Model file for the job. Use its own axes, mm. Face numbers are marked on the shaded views. A direction names the side the tool comes from. Coordinates: 2 decimals unless noted, no trailing zeros. Order: outer loops, then holes, each group sorted by start corner. A loop starts at its lowest first (then second) coordinate and runs counter-clockwise, first axis right, second up. Notation, with made-up numbers: M 4.25,-6.5 L 30.25,-6.5 A30 ccw 30.25,24.5 Z; hole C 54,38 d2. An arc over 180 degrees is marked long. Return JSON: item names as keys, results as strings.
```python
from build123d import *

# Parameters (mm, degrees)
F0_W     = 4.6228
F0_H     = 4.6228
F1_DEPTH = 3.175
F2_DEPTH = 34.925
F3_W     = 4.6228
F3_H     = 4.6228
F4_DEPTH = 25.4


with BuildPart() as f1:
    # F0 (on Front) → F1 (new body)
    with BuildSketch(Plane.XZ):
        Polygon((6.37921, -9.525), (6.37921, 15.875), (-6.37921, 15.875), (-6.37921, -9.525), (-1.8334548599, -9.525), align=None)
        with Locations((-0.02921, -3.175)):
            Rectangle(F0_W, F0_H, mode=Mode.SUBTRACT)
        with Locations((-0.02921, 9.525)):
            Rectangle(F0_W, F0_H, mode=Mode.SUBTRACT)
    extrude(amount=F1_DEPTH)

    # F0 (on Front) → F2 (join)
    with BuildSketch(Plane.XZ):
        Polygon((6.37921, -12.7), (6.37921, -9.525), (-1.8334548599, -9.525), (-6.37921, -9.525), (-6.37921, -12.7), (2.7123002801, -12.7), align=None)
    extrude(amount=F2_DEPTH)

    # F3 (on face) → F4 (cut)
    with BuildSketch(Plane.XY.offset(-9.525)):
        with Locations((0, -14.8336)):
            Rectangle(F3_W, F3_H)
        Polygon((-2.3114, -30.8864), (0, -30.8864), (2.3114, -30.8864), (2.3114, -26.2636), (-2.3114, -26.2636), align=None)
    extrude(amount=-F4_DEPTH, mode=Mode.SUBTRACT)


solid = f1.part
```
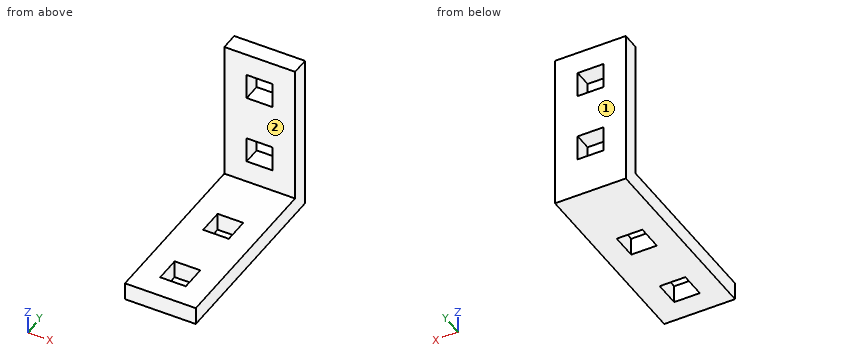
Item 1: Wall check: line 1 (X direction, y = -14.5, z = -10.5); line 2 (Z direction, x = -6, y = -19.5) (3 decimals); line 3 (Y direction, x = -2.5, z = -7) (3 decimals). Give the ranges that are in metal, low to high.
Check result:
{"line 1": "x = -6.38 to -2.31, 2.31 to 6.38", "line 2": "z = -12.7 to -9.525", "line 3": "y = -3.175 to 0"}
Item 2: Saw through at C-C (x = 4.75). Write the cut outline in (y, z) (3 decimals), and give its area (3 significant figures).
Check result:
{"outline": "M -34.925,-12.7 L 0,-12.7 L 0,15.875 L -3.175,15.875 L -3.175,-9.525 L -34.925,-9.525 Z", "area": "192 mm2"}
Item 3: 3-axis set-ups, long thin cutter, end or side, ignore diameter. For the marked faces 1 and 2: which of +Z, -Z, +X, -X, +Y, -Y reach the whole face in a straight line?
Check result:
{"face 1": "+Z, -Z, +X, -X, +Y", "face 2": "+Z, +X, -X, -Y"}
Item 4: Saw through at A-A (x = 0.25). Write the cut outline in (y, z) (3 decimals).
Check result:
{"outline": "M -34.925,-12.7 L -30.886,-12.7 L -30.886,-9.525 L -34.925,-9.525 Z; M -26.264,-12.7 L -17.145,-12.7 L -17.145,-9.525 L -26.264,-9.525 Z; M -12.522,-12.7 L 0,-12.7 L 0,-5.486 L -3.175,-5.486 L -3.175,-9.525 L -12.522,-9.525 Z; M -3.175,-0.864 L 0,-0.864 L 0,7.214 L -3.175,7.214 Z; M -3.175,11.836 L 0,11.836 L 0,15.875 L -3.175,15.875 Z"}
Item 5: Saw through at D-D (y = -24.5). Write the cut outline in (x, z) (3 decimals), and give its area (3 significant figures).
Check result:
{"outline": "M -6.379,-12.7 L 6.379,-12.7 L 6.379,-9.525 L -6.379,-9.525 Z", "area": "40.5 mm2"}
Item 6: Saw through at B-B (z = 11.25). Write the cut outline in (x, y) (3 decimals).
Check result:
{"outline": "M -6.379,-3.175 L -2.341,-3.175 L -2.341,0 L -6.379,0 Z; M 2.282,-3.175 L 6.379,-3.175 L 6.379,0 L 2.282,0 Z"}
Item 7: Drop flat-ended pins along their axis: pin 1 Ø1 at (x, z) = (-3, 3.5) entering from -Y (3 decimals); pin 2 Ø2 at (y, z) = (-16, -7.5) entering from +X; pin 3 Ø3 at (x, y) = (0.5, -16.5) entering from +Z (3 decimals). Give the stop position or say it passes through.
Check result:
{"pin 1": "stops at y = -3.175", "pin 2": "passes through", "pin 3": "stops at z = -9.525"}
